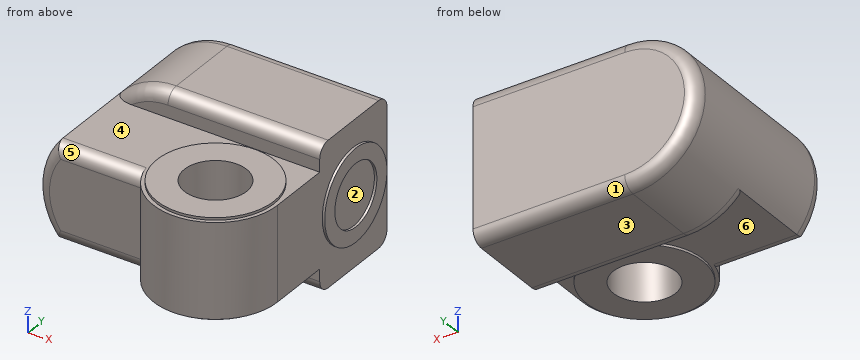
Autodesk Inventor part; units mm, degrees
ref_plane "YZ Plane" through (0, 0, 0) normal (1, 0, 0) x (0, 1, 0)
ref_plane "XZ Plane" through (0, 0, 0) normal (0, 1, 0) x (-1, 0, 0)
ref_plane "XY Plane" through (0, 0, 0) normal (0, 0, 1) x (1, 0, 0)
sketch "Sketch1" plane through (0, 0, 0) normal (0, 1, 0) x (-1, 0, 0)
  line L0 (221.2262, 97.1913) -> (41.2262, 97.1913)
  line L1 (41.2262, 97.1913) -> (41.2262, 213.1913)
  line L2 (41.2262, 213.1913) -> (221.2262, 213.1913)
  line L3 (221.2262, 213.1913) -> (221.2262, 97.1913)
  point P0 (0, 0)
  dimension "d2" = 180
  dimension "d3" = 116
extrude "Extrusion1" add sketch "Sketch1" along normal blind 180
sketch "Sketch2" plane through (-41.2262, 0, 97.1913) normal (0, 0, -1) x (-1, 0, 0)
  point P0 (-41.2262, 0)
sketch "Sketch3" plane through (-41.2262, 0, 213.1913) normal (1, 0, 0) x (0, 0, -1)
  line L0 (0, 0) -> (20, 0)
  line L1 (0, 0) -> (116, 0)
  line L2 (20, 0) -> (96, 0)
  line L3 (20, 0) -> (0, 0)
  line L4 (0, 0) -> (0, 100)
  line L5 (0, 100) -> (20, 100)
  line L6 (20, 100) -> (20, 0)
  line L7 (96, 0) -> (116, 0)
  line L8 (116, 0) -> (116, 100)
  line L9 (116, 100) -> (96, 100)
  line L10 (96, 100) -> (96, 0)
  point P0 (213.1913, 0)
  dimension "d6" = 20
  dimension "d7" = 76
  dimension "d8" = 20
  dimension "d9" = 100
  dimension "d10" = 20
  dimension "d11" = 100
extrude "Extrusion2" cut sketch "Sketch3" against normal blind 200 contours L4 L5 L6 L0
extrude "Extrusion3" cut sketch "Sketch3" against normal blind 200 contours L10 L9 L8 L1
sketch "Sketch4" plane through (-41.2262, 0, 117.1913) normal (0, 0, -1) x (-1, 0, 0)
  circle A0 centre (50, 50) radius 50
  line L0 (180, 0) -> (0, 0)
  line L1 (0, 0) -> (0, 100)
  circle A1 centre (50, 50) radius 47
  line L2 (180, 0) -> (180, 30)
  line L3 (180, 0) -> (180, 100)
  line L4 (180, 30) -> (95.8258, 30)
  point P0 (-41.2262, 0)
  point P1 (0, 50)
  point P2 (50, 0)
  dimension "d16" = 100
  dimension "d17" = 94
  dimension "d29" = 30
extrude "Extrusion4" add sketch "Sketch4" along normal blind 2 contours A1
sketch "Sketch5" plane through (-41.2262, 0, 193.1913) normal (0, 0, 1) x (1, 0, 0)
  circle A0 centre (-50, 50) radius 50
  line L0 (0, 100) -> (0, 0)
  line L1 (0, 0) -> (-180, 0)
  circle A1 centre (-50, 50) radius 47
  point P0 (41.2262, 0)
  dimension "d20" = 100
  dimension "d21" = 94
extrude "Extrusion5" add sketch "Sketch5" along normal blind 2 contours A1
sketch "Sketch6" plane through (-91.2262, 50, 115.1913) normal (0, 0, -1) x (-1, 0, 0)
  circle A0 centre (0, 0) radius 25
  point P0 (-91.2262, -50)
  dimension "d24" = 50
extrude "Extrusion6" cut sketch "Sketch6" against normal blind 200
extrude "Extrusion7" cut sketch "Sketch4" against normal blind 200 contours L0 L1 A0
sketch "Sketch7" plane through (-41.2262, 100, 117.1913) normal (0, 0, -1) x (-1, 0, 0)
  point P0 (-41.2262, -100)
extrude "Extrusion8" cut sketch "Sketch4" against normal blind 200 contours L4 L2 L0 A0
sketch "Sketch8" plane through (0, 180, 0) normal (0, 1, 0) x (1, 0, 0)
  circle A0 centre (-163.2262, -155.1913) radius 58
  line L0 (-221.2262, -97.1913) -> (-221.2262, -213.1913)
  line L1 (-221.2262, -213.1913) -> (-41.2262, -213.1913)
  line L2 (-41.2262, -213.1913) -> (-41.2262, -97.1913)
  line L3 (-221.2262, -213.1913) -> (-41.2262, -213.1913)
  line L4 (-41.2262, -213.1913) -> (-41.2262, -97.1913)
  line L5 (-221.2262, -97.1913) -> (-221.2262, -213.1913)
  line L6 (-221.2262, -97.1913) -> (-41.2262, -97.1913)
  line L7 (-221.2262, -97.1913) -> (-221.2262, -117.1913)
  point P0 (0, 0)
  point P1 (-163.2262, -97.1913)
  point P2 (-221.2262, -155.1913)
  point P3 (-163.2262, -213.1913)
  dimension "d32" = 116
extrude "Extrusion9" cut sketch "Sketch8" against normal blind 200 contours A0 L0 L6
extrude "Extrusion10" cut sketch "Sketch8" against normal blind 200 contours L1 L0 A0
sketch "Sketch10" plane through (-41.2262, 180, 213.1913) normal (1, 0, 0) x (0, 0, -1)
  circle A0 centre (58, -40) radius 37
  circle A1 centre (58, -40) radius 25
  point P0 (213.1913, -180)
  dimension "d39" = 74
  dimension "d40" = 50
extrude "Extrusion11" add sketch "Sketch10" along normal blind 2
fillet "Fillet2" radius 10 2 edges at (-187.3094, 100, 102.4277) (-102.2262, 100, 97.1913)
fillet "Fillet3" radius 10 7 edges at (-102.2262, 100, 213.1913) (-102.2262, 180, 213.1913) (-102.2262, 180, 97.1913) (-221.2262, 180, 155.1913) (-221.2262, 30, 155.1913) (-172.048, 30, 117.1913) (-172.048, 30, 193.1913)
Can you work these out from the model? Positions are in its coordinate system, mm. Face numbers are marked on the shaded views. A direction names the side the tool comes from. Round coordinates to 2 decimals unless told otherwise and drop trailing zeros. Loops run counter-clockwise (first coordinate to the right, second up) from the corner with the lowest first, then second, coordinate; pieces in that order, holes last. Notation, with made-up numbers: (24, 40.5) - (36, 40.5) arc R19 ccw to (36, 54.5) - close; hole circle Ø10 at (-24.75, 7.25). An arc over 180 degrees is marked (long way). Answer in a Markdown table with one row per item. Add a question column.
Q1. For pin 1 Ø10 at (x, z) = (-154.5, 186.5) entering from -Y; pin 2 Ø8 at (x, y) = (-183.5, 125) entering from -Z; pin 3 Ø3 at (x, y) = (-98, 109.5) entering from -Z; pin 4 Ø8 at (x, y) = (-175, 155) entering from +Z, each with a flat end and sliding along its axis, tell me the tip position at first contact or that it passes through.
Q2. I want a section at A-A on x = -144.5. List the corners of the cut face in (y, z) for me.
Q3. I want a section at B-B on y = 140. List the corners of the cut face in (x, z) for me.
Q4. We'd pull the mould along Y, two halves only. Please class the marked faces 1, 2 and 3: pulls with the +Y half, pulls with the -Y half, needs draft (parallel to the pull), parting line crosses it, or undercut.
Q5. I want a section at C-C on x = -80.5. List the corners of the cut face in (y, z) for me.
Q6. I need wall thicknesses on L1, parallel to Y at x = -114, z = 193.5; L2, parallel to Y at x = -200, z = 130.5; L3, parallel to Y at x = -112.5, z = 182.5. Which ranges of each line are inside material? Lowest first, please.
Q7. Which directions (+Z, -Z, +X, -X, +Y, -Y) give clear straight access to the entire face, cutting with the end or side of a thin tool? Please do the marked faces 4, 5 and 6.
Q8. I want a section at D-D on y = 94. List the corners of the cut face in (x, z) for me.
A:
| question | item | result |
|---|---|---|
| 1 | pin 1 | y = 30 |
| 1 | pin 2 | z = 99.52 |
| 1 | pin 3 | z = 97.19 |
| 1 | pin 4 | z = 212.67 |
| 2 | outline | (30, 127.19) arc R10 ccw to (40, 117.19) - (100, 117.19) - (100, 107.19) arc R10 ccw to (110, 97.19) - (170, 97.19) arc R10 ccw to (180, 107.19) - (180, 203.19) arc R10 ccw to (170, 213.19) - (110, 213.19) arc R10 ccw to (100, 203.19) - (100, 193.19) - (40, 193.19) arc R10 ccw to (30, 183.19) - close |
| 3 | outline | (-163.23, 97.19) - (-41.23, 97.19) - (-41.23, 118.19) - (-39.23, 118.19) - (-39.23, 130.19) - (-41.23, 130.19) - (-41.23, 180.19) - (-39.23, 180.19) - (-39.23, 192.19) - (-41.23, 192.19) - (-41.23, 213.19) - (-163.23, 213.19) arc R58 ccw to start |
| 4 | face 1 | pulls with the +Y half |
| 4 | face 2 | undercut |
| 4 | face 3 | needs draft |
| 5 | outline | (1.16, 117.19) - (4.24, 117.19) - (4.24, 115.19) - (27.42, 115.19) - (27.42, 195.19) - (4.24, 195.19) - (4.24, 193.19) - (1.16, 193.19) - close; (72.58, 115.19) - (95.76, 115.19) - (95.76, 117.19) - (100, 117.19) - (100, 107.19) arc R10 ccw to (110, 97.19) - (170, 97.19) arc R10 ccw to (180, 107.19) - (180, 203.19) arc R10 ccw to (170, 213.19) - (110, 213.19) arc R10 ccw to (100, 203.19) - (100, 193.19) - (95.76, 193.19) - (95.76, 195.19) - (72.58, 195.19) - close |
| 6 | L1 | 8.89 to 39.69, 60.31 to 91.11, 100 to 180 |
| 6 | L2 | 30 to 180 |
| 6 | L3 | 4.75 to 36.87, 63.13 to 180 |
| 7 | face 4 | +Z |
| 7 | face 5 | +Z, -X, -Y |
| 7 | face 6 | -Z |
| 8 | outline | (-207.04, 117.19) - (-107.75, 117.19) - (-107.75, 115.19) - (-74.7, 115.19) - (-74.7, 117.19) - (-41.23, 117.19) - (-41.23, 193.19) - (-74.7, 193.19) - (-74.7, 195.19) - (-107.75, 195.19) - (-107.75, 193.19) - (-207.04, 193.19) arc R58 ccw to start |
